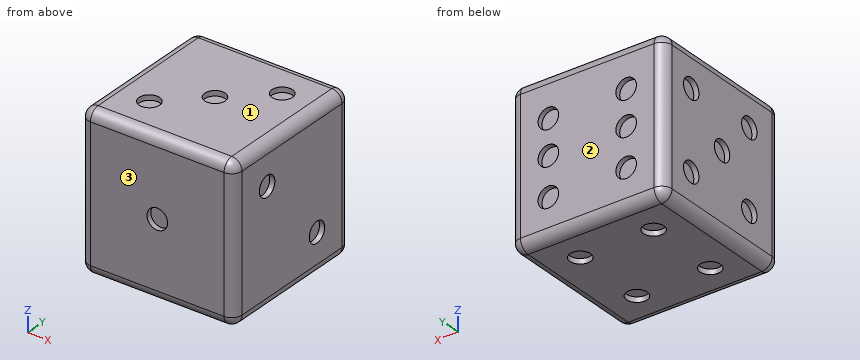
```python
from build123d import *

# Parameters (mm, degrees)
F0_W      = 15
F0_H      = 15
F1_DEPTH  = 15
F2_R      = 1
F4_DEPTH  = 0.5
F5_R      = 1
F6_DEPTH  = 0.5
F7_R      = 1
F8_DEPTH  = 0.5
F9_R      = 1
F10_DEPTH = 0.5
F11_R     = 1
F12_DEPTH = 0.5
F13_R     = 1
F14_DEPTH = 0.5
F15_R     = 1


with BuildPart() as f1:
    # F0 (on Front) → F1 (new body)
    with BuildSketch(Plane.XZ):
        Rectangle(F0_W, F0_H)
    extrude(amount=F1_DEPTH)

    # F2 (on face) → F4 (cut)
    with BuildSketch(Plane.XZ.offset(15)):
        Circle(F2_R)
    extrude(amount=-F4_DEPTH, mode=Mode.SUBTRACT)

    # F5 (on face) → F6 (cut)
    with BuildSketch(Plane(origin=(0, 0, 0), x_dir=(-1, 0, 0), z_dir=(0, 1, 0))):
        with Locations((3.785098, -3.737234)):
            Circle(F5_R)
        with Locations((3.785098, 0)):
            Circle(F5_R)
        with Locations((3.785098, 3.375805)):
            Circle(F5_R)
        with Locations((-3.786711, -3.737234)):
            Circle(F5_R)
        with Locations((-3.786711, 0)):
            Circle(F5_R)
        with Locations((-3.786711, 3.375805)):
            Circle(F5_R)
    extrude(amount=-F6_DEPTH, mode=Mode.SUBTRACT)

    # F7 (on face) → F8 (cut)
    with BuildSketch(Plane(origin=(0, 0, -7.5), x_dir=(1, 0, 0), z_dir=(0, 0, -1))):
        with Locations((3.532658, 3.806027)):
            Circle(F7_R)
        with Locations((3.532658, 11.167861)):
            Circle(F7_R)
        with Locations((-3.600359, 3.806027)):
            Circle(F7_R)
        with Locations((-3.600359, 11.167861)):
            Circle(F7_R)
    extrude(amount=-F8_DEPTH, mode=Mode.SUBTRACT)

    # F9 (on face) → F10 (cut)
    with BuildSketch(Plane(origin=(-7.5, 0, 0), x_dir=(0, -1, 0), z_dir=(-1, 0, 0))):
        with Locations((7.5, 0)):
            Circle(F9_R)
        with Locations((3.496341, -3.811767)):
            Circle(F9_R)
        with Locations((11.03965, -3.811767)):
            Circle(F9_R)
        with Locations((11.03965, 3.736319)):
            Circle(F9_R)
        with Locations((3.496341, 3.736319)):
            Circle(F9_R)
    extrude(amount=-F10_DEPTH, mode=Mode.SUBTRACT)

    # F11 (on face) → F12 (cut)
    with BuildSketch(Plane.YZ.offset(7.5)):
        with Locations((-4.266871, -3.594229)):
            Circle(F11_R)
        with Locations((-10.73485, 3.598094)):
            Circle(F11_R)
    extrude(amount=-F12_DEPTH, mode=Mode.SUBTRACT)

    # F13 (on face) → F14 (cut)
    with BuildSketch(Plane.XY.offset(7.5)):
        with Locations((3.862818, -3.929111)):
            Circle(F13_R)
        with Locations((0, -7.5)):
            Circle(F13_R)
        with Locations((-3.697416, -11.085594)):
            Circle(F13_R)
    extrude(amount=-F14_DEPTH, mode=Mode.SUBTRACT)

    # F15
    f15_edges = [f1.edges().sort_by_distance(p)[0] for p in [
        (7.5, 0, 0),
        (0, 0, -7.5),
        (7.5, -7.5, -7.5),
        (-7.5, 0, 0),
        (0, 0, 7.5),
        (-7.5, -7.5, 7.5),
        (7.5, -7.5, 7.5),
        (0, -15, 7.5),
        (-7.5, -15, 0),
        (-7.5, -7.5, -7.5),
        (7.5, -15, 0),
        (0, -15, -7.5),
    ]]
    fillet(f15_edges, radius=F15_R)


solid = f1.part
```
Verification items for the finished model (mm, model axes). Face numbers are marked on the shaded views. Coordinates: 2 decimals unless noted, no trailing zeros. Write each loop counter-clockwise with the first axis right and the second up, starting at its lowest first coordinate (ties: lowest second). Pieces come first, ordered by that corner, then holes. Notation, with made-up numbers: M 75.25,45 L 80.25,45 A20 ccw 80.25,84 Z; hole C 27.25,-39.75 d10. An arc over 180 degrees is marked long. One line per item, written item: value.
Item 1: Mould release check, pull along Y, two halves, no side actions. Record for the marked faces 1, 2 and 3: pulls with the +Y half, pulls with the -Y half, needs draft (parallel to the pull), parting line crosses it, or undercut.
Check sheet entries:
face 1: needs draft
face 2: pulls with the +Y half
face 3: pulls with the -Y half
Item 2: Section check A-A, the plane z = 0. Record the boundary of the cut face in (x, y), plus the area to 3 significant figures.
Check sheet entries:
outline: M -7.5,-14 A1 ccw -6.5,-15 L -1,-15 L -1,-14.5 L 1,-14.5 L 1,-15 L 6.5,-15 A1 ccw 7.5,-14 L 7.5,-1 A1 ccw 6.5,0 L 4.79,0 L 4.79,-0.5 L 2.79,-0.5 L 2.79,0 L -2.79,0 L -2.79,-0.5 L -4.79,-0.5 L -4.79,0 L -6.5,0 A1 ccw -7.5,-1 L -7.5,-6.5 L -7,-6.5 L -7,-8.5 L -7.5,-8.5 Z
area: 220 mm^2
Item 3: Gauge pin test, flat ends, axial feed: pin 1 Ø1 at (y, z) = (-10.5, 3.5) entering from +X; pin 2 Ø1.6 at (x, z) = (-3.79, -3.74) entering from +Y; pin 3 Ø0.6 at (y, z) = (-4, -3.5) entering from -X. Record the tip position at first contact, or that the pin passes through.
Check sheet entries:
pin 1: stops at x = 7
pin 2: stops at y = -0.5
pin 3: stops at x = -7
Item 4: Scan lines: line 1 along X through (y, z) = (-10.5, 3.75); line 2 along X through (y, z) = (-11.5, -3.75); line 3 along Y through (x, z) = (-4.5, 0). Record each from-to range of solid material in increasing order.
Check sheet entries:
line 1: x = -7 to 7
line 2: x = -7 to 7.5
line 3: y = -15 to -0.5
